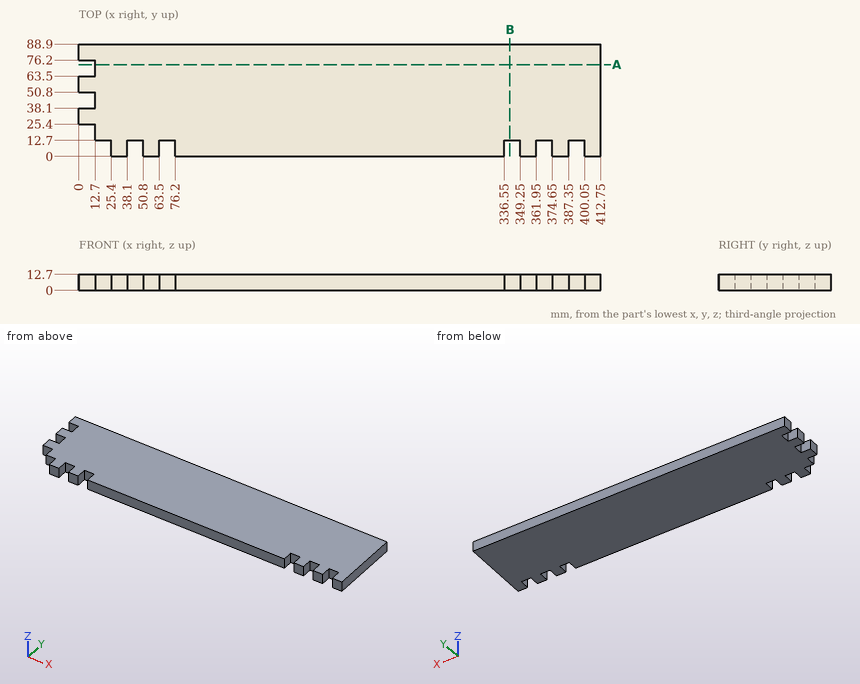
Can you work these out from the drawing? Everything is in mm from the part's minimum corner. Round coordinates to 2 decimals unless told otherwise and drop trailing zeros. Write each loop counter-clockwise with the first axis right and the second up, starting at its lowest first coordinate (ties: lowest second). Pieces come first, ordered by that corner, then holes. Notation, with made-up numbers: (82, 72.5) - (94, 72.5) arc R21 ccw to (94, 92.5) - close; hole circle Ø9 at (31, 53.5). An arc over 180 degrees is marked (long way). Put each result on its own line as item: value. Start each with the question number.
(1) I need wall thicknesses on probe 1 along X at (y, z) = (5.5, 6); probe 2 along X at (y, z) = (42, 7.25). Which ranges of each line are inside material? Lowest first, please.
(2) I want a section at B-B, the plane x = 341. Please give me the cut outline in (y, z).
(3) I want a section at A-A, the plane y = 72.5. Please give me the cut outline in (x, z), plus the area to 3 significant figures.
(4) Will these pins go through, and if not, where does the flat tip stop? pin 1 (6.5 mm diameter, centred on y = 5, z = 3.5, fed in from -X); pin 2 (6.5 mm diameter, centred on x = 47.5, z = 5, fed in from -Y).
Here are the results:
1. probe 1: x = 25.4 to 38.1, 50.8 to 63.5, 76.2 to 336.55, 349.25 to 361.95, 374.65 to 387.35, 400.05 to 412.75
1. probe 2: x = 12.7 to 412.75
2. outline: (12.7, 0) - (88.9, 0) - (88.9, 12.7) - (12.7, 12.7) - close
3. outline: (12.7, 0) - (412.75, 0) - (412.75, 12.7) - (12.7, 12.7) - close
3. area: 5,080 mm^2
4. pin 1: stops at x = 25.4
4. pin 2: stops at y = 12.7
